```python
from build123d import *

# Parameters (mm, degrees)
SKETCH1_W           = 215
SKETCH1_H           = 18
SKETCH1_R           = 3
BOSS_EXTRUDE1_DEPTH = 20
SKETCH1_3_W         = 80
SKETCH1_3_H         = 18
SKETCH1_3_R         = 3
BOSS_EXTRUDE2_DEPTH = 47
BOSS_EXTRUDE3_START = 47
SKETCH1_6_W         = 25
SKETCH1_6_H         = 18
SKETCH1_6_W_2       = 27.5
SKETCH1_6_R         = 3
BOSS_EXTRUDE3_DEPTH = 10
SKETCH2_R           = 6.975
SKETCH2_R_2         = 4.475
SKETCH2_R_3         = 3
BOSS_EXTRUDE4_DEPTH = 25
SKETCH2_6_R         = 10.5
SKETCH2_6_R_2       = 3
SKETCH2_6_W         = 9.3
SKETCH2_6_H         = 5
CUT_EXTRUDE5_DEPTH  = 224.828059035
SKETCH1_8_R         = 3
CUT_EXTRUDE6_DEPTH  = 57
CHAMFER1_SIZE       = 37.320508076
CHAMFER1_SIZE_2     = 10
CHAMFER2_SIZE       = 10
CHAMFER2_SIZE_2     = 37.320508076


with BuildPart() as part:
    # Sketch1 → Boss-Extrude1 (new body)
    with BuildSketch(Plane(origin=(0, 0, 0), x_dir=(1, 0, 0), z_dir=(0, 1, 0))):
        with Locations((107.5, -9)):
            Rectangle(SKETCH1_W, SKETCH1_H)
        with Locations(Location((9.99, -11.15, 0), (0, 0, 270))):
            Circle(SKETCH1_R, mode=Mode.SUBTRACT)
        with Locations(Location((41.99, -11.15, 0), (0, 0, 270))):
            Circle(SKETCH1_R, mode=Mode.SUBTRACT)
        with Locations(Location((79.5033, -10.15, 0), (0, 0, 270))):
            Circle(SKETCH1_R, mode=Mode.SUBTRACT)
        with Locations(Location((135.5033, -10.15, 0), (0, 0, 270))):
            Circle(SKETCH1_R, mode=Mode.SUBTRACT)
        with Locations(Location((173.0133, -11.15, 0), (0, 0, 270))):
            Circle(SKETCH1_R, mode=Mode.SUBTRACT)
        with Locations(Location((205.0133, -11.15, 0), (0, 0, 270))):
            Circle(SKETCH1_R, mode=Mode.SUBTRACT)
    extrude(amount=BOSS_EXTRUDE1_DEPTH)

    # Sketch1<3> → Boss-Extrude2 (add)
    with BuildSketch(Plane(origin=(0, 0, 0), x_dir=(1, 0, 0), z_dir=(0, 1, 0))):
        with Locations((107.5033, -9)):
            Rectangle(SKETCH1_3_W, SKETCH1_3_H)
        with Locations((79.5033, -10.15)):
            Circle(SKETCH1_3_R, mode=Mode.SUBTRACT)
        with Locations((135.5033, -10.15)):
            Circle(SKETCH1_3_R, mode=Mode.SUBTRACT)
    extrude(amount=BOSS_EXTRUDE2_DEPTH)

    # Sketch1<6> → Boss-Extrude3 (add)
    # profile 1 of 3: a face of its own
    with BuildSketch(Plane(origin=(0, 0, 0), x_dir=(1, 0, 0), z_dir=(0, 1, 0)).offset(BOSS_EXTRUDE3_START)):
        with Locations((107.5033, -9)):
            Rectangle(SKETCH1_6_W, SKETCH1_6_H)
        with BuildLine():
            ThreePointArc((111.0033, -10.75), (107.5033, -14.25), (104.0033, -10.75))
            Line((104.0033, -10.75), (104.0033, -7.25))
            ThreePointArc((104.0033, -7.25), (107.5033, -3.75), (111.0033, -7.25))
            Line((111.0033, -7.25), (111.0033, -10.75))
        make_face(mode=Mode.SUBTRACT)
    # profile 2 of 3: a face of its own
    with BuildSketch(Plane(origin=(0, 0, 0), x_dir=(1, 0, 0), z_dir=(0, 1, 0)).offset(BOSS_EXTRUDE3_START)):
        with Locations((81.2533, -9)):
            Rectangle(SKETCH1_6_W_2, SKETCH1_6_H)
        with Locations(Location((79.5033, -10.15, 0), (0, 0, 270))):
            Circle(SKETCH1_6_R, mode=Mode.SUBTRACT)
    # profile 3 of 3: a face of its own
    with BuildSketch(Plane(origin=(0, 0, 0), x_dir=(1, 0, 0), z_dir=(0, 1, 0)).offset(BOSS_EXTRUDE3_START)):
        with Locations((133.7533, -9)):
            Rectangle(SKETCH1_6_W_2, SKETCH1_6_H)
        with Locations(Location((135.5033, -10.15, 0), (0, 0, 270))):
            Circle(SKETCH1_6_R, mode=Mode.SUBTRACT)
    extrude(amount=BOSS_EXTRUDE3_DEPTH)

    # Sketch2 → Boss-Extrude4 (add)
    # profile 1 of 4: a face of its own
    with BuildSketch(Plane.XY.offset(18)):
        with Locations((87.5033, 38.99)):
            Circle(SKETCH2_R)
        with Locations((87.5033, 38.99)):
            Circle(SKETCH2_R_2, mode=Mode.SUBTRACT)
    # profile 2 of 4: a face of its own
    with BuildSketch(Plane.XY.offset(18)):
        with Locations((87.5033, 38.99)):
            Circle(SKETCH2_R_2)
        with Locations((87.5033, 38.99)):
            Circle(SKETCH2_R_3, mode=Mode.SUBTRACT)
    # profile 3 of 4: a face of its own
    with BuildSketch(Plane.XY.offset(18)):
        with Locations((127.5033, 38.99)):
            Circle(SKETCH2_R)
        with Locations((127.5033, 38.99)):
            Circle(SKETCH2_R_2, mode=Mode.SUBTRACT)
    # profile 4 of 4: a face of its own
    with BuildSketch(Plane.XY.offset(18)):
        with Locations((127.5033, 38.99)):
            Circle(SKETCH2_R_2)
        with Locations((127.5033, 38.99)):
            Circle(SKETCH2_R_3, mode=Mode.SUBTRACT)
    extrude(amount=-BOSS_EXTRUDE4_DEPTH)

    # Sketch2<6> → Cut-Extrude5 (cut, through all)
    with BuildSketch(Plane.XY.offset(18)):
        with Locations((107.5033, 39.05)):
            Circle(SKETCH2_6_R)
        with Locations((87.5033, 38.99)):
            Circle(SKETCH2_6_R_2)
        with Locations((79.5033, 28.5)):
            Rectangle(SKETCH2_6_W, SKETCH2_6_H)
        with Locations((127.5033, 38.99)):
            Circle(SKETCH2_6_R_2)
        with Locations((135.5033, 28.5)):
            Rectangle(SKETCH2_6_W, SKETCH2_6_H)
    extrude(amount=-CUT_EXTRUDE5_DEPTH, mode=Mode.SUBTRACT)

    # Sketch1<8> → Cut-Extrude6 (cut)
    with BuildSketch(Plane(origin=(0, 0, 0), x_dir=(1, 0, 0), z_dir=(0, 1, 0))):
        with Locations(Location((135.5033, -10.15, 0), (0, 0, 180))):
            Circle(SKETCH1_8_R)
        with Locations(Location((79.5033, -10.15, 0), (0, 0, 270))):
            Circle(SKETCH1_8_R)
    extrude(amount=CUT_EXTRUDE6_DEPTH, mode=Mode.SUBTRACT)

    # Chamfer1
    # the kernel refuses this chamfer: 37.320508076, 10 mm, written as the material it adds along each edge
    with BuildSketch(Plane(origin=(147.5033, 20, 18), x_dir=(-0.009967146577156421, 0.9999503267608394, 0), z_dir=(0, 0, -1))) as chamfer1_piece_1_section:
        Polygon((CHAMFER1_SIZE * 0.999950326753, CHAMFER1_SIZE * 0.00996714657707), (-CHAMFER1_SIZE_2 * 0.00996714657716, CHAMFER1_SIZE_2 * 0.999950326761), (0, 0), align=None)
    chamfer1_piece_1 = extrude(amount=18, mode=Mode.PRIVATE)
    chamfer1_piece_1 = split(chamfer1_piece_1, bisect_by=Plane(origin=(150.477287082, 57, 9), z_dir=(0, -1, 0)), keep=Keep.TOP, mode=Mode.PRIVATE)
    add(chamfer1_piece_1)

    # Chamfer2
    # the kernel refuses this chamfer: 37.320508076, 10 mm, written as the material it adds along each edge
    with BuildSketch(Plane(origin=(67.5033, 20, 0), x_dir=(-0.9905000388259542, -0.137512447021291, 0), z_dir=(0, 0, 1))) as chamfer2_piece_1_section:
        Polygon((CHAMFER2_SIZE * 0.990500038826, -CHAMFER2_SIZE * 0.137512447021), (-CHAMFER2_SIZE_2 * 0.13751244702, -CHAMFER2_SIZE_2 * 0.990500038818), (0, 0), align=None)
    chamfer2_piece_1 = extrude(amount=18, mode=Mode.PRIVATE)
    chamfer2_piece_1 = split(chamfer2_piece_1, bisect_by=Plane(origin=(64.529312918, 57, 9), z_dir=(0, -1, 0)), keep=Keep.TOP, mode=Mode.PRIVATE)
    add(chamfer2_piece_1)


solid = part.part
```
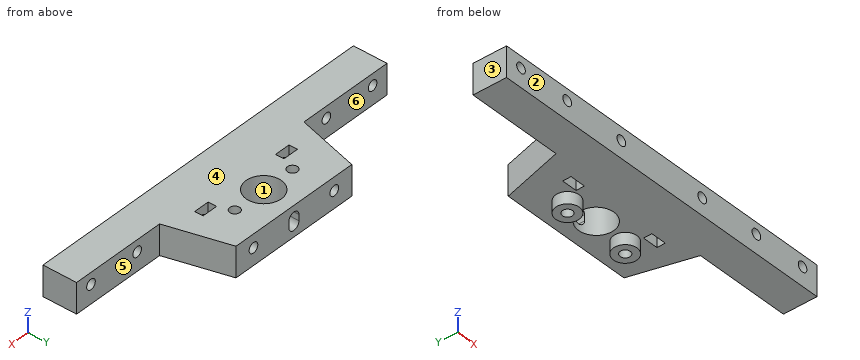
Verification items for the finished model (mm, model axes). Face numbers are marked on the shaded views. A direction names the side the tool comes from. Round coordinates to 2 decimals unless told otherwise and drop trailing zeros. Order: outer loops, then holes, each group sorted by start corner. A loop starts at its lowest first (then second) coordinate and runs counter-clockwise, first axis right, second up. Notation, with made-up numbers: (-39, 55.25) - (-7, 55.25) arc R15 ccw to (-7, 71.25) - close; hole circle Ø9 at (-33.75, 85). An arc over 180 degrees is marked (long way). Use CSV: the item, a comma, the result in double quotes. Start each with the question number.
1) Section check C-C, the plane x = 145. Record the cut outline in (y, z), plus the area to 3 significant figures.
2) Section check A-A, the plane x = 9.99. Record the cut outline in (y, z), plus the area to 3 significant figures.
3) Mould release check, pull along Y, two halves, no side actions. Record for the marked faces 1, 2 and 3: +Y half, -Y half, draft (parallel to the pull), parting line (faces both ways), or undercut.
4) Section check B-B, the plane y = 15. Record the cut outline in (x, z), plus the area to 3 significant figures.
5) Thickness scan on L1, parallel to Z at x = 80, y = 35.5; L2, parallel to X at y = 52.5, z = 12; L3, parallel to X at y = 35, z = 10.25. Record the ranges inside material, lowest first.
6) Access from +Z, -Z, +X, -X, +Y, -Y to the whole of each face (thin tool, end or side, straight path). Record for the marked faces 4, 5 and 6.
7) Go/stop test with flat-tipped pins: P1, Ø2.5, axis at y = 28.5, z = 12, coming from the -X side; P2, Ø1, axis at y = 52, z = 9.5, coming from the -X side; P3, Ø14.5, axis at x = 185, z = 8.5, coming from the +Y side. Record where each tip stops, or that it passes through.
Answers:
1,outline,"(0, 0) - (57, 0) - (57, 18) - (0, 18) - close"
1,area,"1,030 mm²"
2,outline,"(0, 0) - (20, 0) - (20, 8.15) - (0, 8.15) - close; (0, 14.15) - (20, 14.15) - (20, 18) - (0, 18) - close"
2,area,"240 mm²"
3,face 1,"undercut"
3,face 2,"-Y half"
3,face 3,"draft"
4,outline,"(0, 0) - (215, 0) - (215, 18) - (0, 18) - close; hole circle Ø6 at (9.99, 11.15); hole circle Ø6 at (41.99, 11.15); hole circle Ø6 at (79.5, 10.15); hole circle Ø6 at (135.5, 10.15); hole circle Ø6 at (173.01, 11.15); hole circle Ø6 at (205.01, 11.15)"
4,area,"3,700 mm²"
5,L1,"z = 0 to 7.19, 13.11 to 18"
5,L2,"x = 66.21 to 77.14, 81.86 to 104.23, 110.77 to 133.14, 137.86 to 148.79"
5,L3,"x = 61.52 to 76.5, 82.5 to 97.82, 117.19 to 132.5, 138.5 to 153.48"
6,face 4,"+Z, +X, -X, +Y, -Y"
6,face 5,"+Z, -Z, +X, +Y"
6,face 6,"+Z, -Z, -X, +Y"
7,P1,"stops at x = 59.45"
7,P2,"stops at x = 65.94"
7,P3,"stops at y = 20"
